from build123d import *

# Parameters (mm, degrees)
SKETCH1_W           = 80
SKETCH1_H           = 225
BOSS_EXTRUDE1_DEPTH = 29
CUT_EXTRUDE1_REACH  = 124.871
SKETCH4_R           = 10
CUT_EXTRUDE2_DEPTH  = 17
SKETCH5_R           = 8.5
CUT_EXTRUDE3_DEPTH  = 5
CUT_EXTRUDE4_REACH  = 124.871
SKETCH6_W           = 12
SKETCH6_H           = 11.5
M10_TAPPED_HOLE1_D  = 8.5
CUT_EXTRUDE5_REACH  = 124.871
SKETCH10_R          = 4


with BuildPart() as part:
    # Sketch1 → Boss-Extrude1 (new body)
    with BuildSketch(Plane(origin=(0, 0, 0), x_dir=(1, 0, 0), z_dir=(0, 1, 0))):
        Rectangle(SKETCH1_W, SKETCH1_H)
    extrude(amount=-BOSS_EXTRUDE1_DEPTH)

    # Sketch2 → Cut-Extrude1 (cut, up to next)
    with BuildSketch(Plane(origin=(0, 0, 0), x_dir=(1, 0, 0), z_dir=(0, 1, 0)), mode=Mode.PRIVATE) as cut_extrude1_sk1:
        with BuildLine():
            Line((-19, 36.36), (-19, 53.86))
            ThreePointArc((-19, 53.86), (-21.5, 56.36), (-24, 53.86))
            Line((-24, 53.86), (-24, 36.36))
            ThreePointArc((-24, 36.36), (-21.5, 33.86), (-19, 36.36))
        make_face()
    cut_extrude1_tool1 = extrude(cut_extrude1_sk1.sketch, amount=-CUT_EXTRUDE1_REACH, mode=Mode.PRIVATE) & part.part
    # Sketch2 → Cut-Extrude1 (cut, up to next)
    with BuildSketch(Plane(origin=(0, 0, 0), x_dir=(1, 0, 0), z_dir=(0, 1, 0)), mode=Mode.PRIVATE) as cut_extrude1_sk2:
        with BuildLine():
            Line((-19, -36.59), (-19, -16.59))
            ThreePointArc((-19, -16.59), (-21.5, -14.09), (-24, -16.59))
            Line((-24, -16.59), (-24, -36.59))
            ThreePointArc((-24, -36.59), (-21.5, -39.09), (-19, -36.59))
        make_face()
    cut_extrude1_tool2 = extrude(cut_extrude1_sk2.sketch, amount=-CUT_EXTRUDE1_REACH, mode=Mode.PRIVATE) & part.part
    # Sketch2 → Cut-Extrude1 (cut, up to next)
    with BuildSketch(Plane(origin=(0, 0, 0), x_dir=(1, 0, 0), z_dir=(0, 1, 0)), mode=Mode.PRIVATE) as cut_extrude1_sk3:
        with BuildLine():
            Line((24, 17.36), (24, 34.86))
            ThreePointArc((24, 34.86), (21.5, 37.36), (19, 34.86))
            Line((19, 34.86), (19, 17.36))
            ThreePointArc((19, 17.36), (21.5, 14.86), (24, 17.36))
        make_face()
    cut_extrude1_tool3 = extrude(cut_extrude1_sk3.sketch, amount=-CUT_EXTRUDE1_REACH, mode=Mode.PRIVATE) & part.part
    # Sketch2 → Cut-Extrude1 (cut, up to next)
    with BuildSketch(Plane(origin=(0, 0, 0), x_dir=(1, 0, 0), z_dir=(0, 1, 0)), mode=Mode.PRIVATE) as cut_extrude1_sk4:
        with BuildLine():
            Line((24, -36.64), (24, -12.64))
            ThreePointArc((24, -12.64), (21.5, -10.14), (19, -12.64))
            Line((19, -12.64), (19, -36.64))
            ThreePointArc((19, -36.64), (21.5, -39.14), (24, -36.64))
        make_face()
    cut_extrude1_tool4 = extrude(cut_extrude1_sk4.sketch, amount=-CUT_EXTRUDE1_REACH, mode=Mode.PRIVATE) & part.part
    add(cut_extrude1_tool1.solids().sort_by_distance((-21.5, 0, -45.11))[0], mode=Mode.SUBTRACT)
    add(cut_extrude1_tool2.solids().sort_by_distance((-21.5, 0, 26.59))[0], mode=Mode.SUBTRACT)
    add(cut_extrude1_tool3.solids().sort_by_distance((21.5, 0, -26.11))[0], mode=Mode.SUBTRACT)
    add(cut_extrude1_tool4.solids().sort_by_distance((21.5, 0, 24.64))[0], mode=Mode.SUBTRACT)

    # Sketch4 → Cut-Extrude2 (cut)
    with BuildSketch(Plane(origin=(0, 0, 0), x_dir=(1, 0, 0), z_dir=(0, 1, 0))):
        with Locations(Location((-22, 72, 0), (0, 0, 270))):
            Circle(SKETCH4_R)
        with Locations(Location((22, 60, 0), (0, 0, 270))):
            Circle(SKETCH4_R)
        with Locations(Location((0, 35, 0), (0, 0, 270))):
            Circle(SKETCH4_R)
        with Locations(Location((0, -25, 0), (0, 0, 270))):
            Circle(SKETCH4_R)
        with Locations(Location((22, -55, 0), (0, 0, 270))):
            Circle(SKETCH4_R)
        with Locations(Location((-22, -55, 0), (0, 0, 270))):
            Circle(SKETCH4_R)
    extrude(amount=-CUT_EXTRUDE2_DEPTH, mode=Mode.SUBTRACT)

    # Sketch5 → Cut-Extrude3 (cut)
    with BuildSketch(Plane.XZ.offset(29)):
        with Locations(Location((0, 100, 0), (0, 0, 270))):
            Circle(SKETCH5_R)
        with Locations(Location((0, -100, 0), (0, 0, 270))):
            Circle(SKETCH5_R)
    extrude(amount=-CUT_EXTRUDE3_DEPTH, mode=Mode.SUBTRACT)

    # Sketch6 → Cut-Extrude4 (cut, up to next)
    with BuildSketch(Plane(origin=(0, 0, 0), x_dir=(1, 0, 0), z_dir=(0, 1, 0)), mode=Mode.PRIVATE) as cut_extrude4_sk1:
        with Locations((23.25, -106.75)):
            Rectangle(SKETCH6_W, SKETCH6_H)
    cut_extrude4_tool1 = extrude(cut_extrude4_sk1.sketch, amount=-CUT_EXTRUDE4_REACH, mode=Mode.PRIVATE) & part.part
    add(cut_extrude4_tool1.solids().sort_by_distance((23.25, 0, 106.75))[0], mode=Mode.SUBTRACT)

    # M10 Tapped Hole1 (through all)
    with Locations(Plane(origin=(0, 0, 0), x_dir=(1, 0, 0), z_dir=(0, 1, 0))):
        with Locations((0, -77.5), (30, 4), (-30, 4), (0, 77.5)):
            Hole(M10_TAPPED_HOLE1_D / 2)

    # Sketch10 → Cut-Extrude5 (cut, up to next)
    with BuildSketch(Plane(origin=(0, 0, 0), x_dir=(1, 0, 0), z_dir=(0, 1, 0)), mode=Mode.PRIVATE) as cut_extrude5_sk1:
        with Locations(Location((0, 9.86, 0), (0, 0, 270))):
            Circle(SKETCH10_R)
    cut_extrude5_tool1 = extrude(cut_extrude5_sk1.sketch, amount=-CUT_EXTRUDE5_REACH, mode=Mode.PRIVATE) & part.part
    add(cut_extrude5_tool1.solids().sort_by_distance((0, 0, -9.86))[0], mode=Mode.SUBTRACT)


solid = part.part
Here's how the part is built. I have some questions about the finished solid (model axes, mm). A direction names the side the tool comes from. Coordinates: 2 decimals unless noted, no trailing zeros. Order: outer loops, then holes, each group sorted by start corner. A loop starts at its lowest first (then second) coordinate and runs counter-clockwise, first axis right, second up. Notation, with made-up numbers: M -12,-35.75 L 2,-35.75 A21 cw 2,-26.75 Z; hole C 51.25,58.25 d6. An arc over 180 degrees is marked long. Answer as CSV lines item,"result".
Item 1: For pin 1 (16 mm diameter, centred on x = -3, z = -40, fed in from +Y); pin 2 (7 mm diameter, centred on x = -30, z = -4, fed in from -Y); pin 3 (10 mm diameter, centred on x = 0, z = 100, fed in from -Y); pin 4 (6 mm diameter, centred on x = 20, z = -60, fed in from +Y), each with a flat end and sliding along its axis, tell me the tip position at first contact or that it passes through.
Results found:
pin 1,"y = 0"
pin 2,"through"
pin 3,"y = -24"
pin 4,"y = -17"
Item 2: Imagine slicing it at C-C on z = -60. Write out the boundary of the cut face in (x, y).
Results found:
outline,"M -40,-29 L 40,-29 L 40,0 L 32,0 L 32,-17 L 12,-17 L 12,0 L -40,0 Z"
Item 3: Imagine slicing it at A-A on y = -26.5. Give the number of separate pieces and of enclosed holes in the cut face, plus the area to 3 significant figures.
Results found:
separate pieces,"1"
enclosed holes,"11"
area,"16,700 mm2"
Item 4: On a 3-axis mill with a long thin cutter (end or side, diameter ignored), from which of +Z, -Z, +X, -X, +Y, -Y can I reach the whole of each face in a straight line? I mean faces 1 (the face through (-21.45, -14.3, 14.09)), 2 (the face through (0, -8, -45)), 3 (the face through (0.37, -26.54, -91.51)). Say none if no direction works.
Results found:
face 1,"+Y, -Y"
face 2,"+Y"
face 3,"-Y"
Item 5: We'd pull the mould along X, two halves only. Please class faces 4 (the face through (21.55, -14.3, -37.36)), 5 (the face through (-1, -29, -2)), 6 (the face through (-40, -14, 2)): +X half, -X half, draft (parallel to the pull), parting line (faces both ways), or undercut.
Results found:
face 4,"undercut"
face 5,"draft"
face 6,"-X half"
Item 6: Imagine slicing it at B-B on x = -30. Write out the boundary of the cut face in (y, z).
Results found:
outline,"M -29,-112.5 L 0,-112.5 L 0,-78 L -17,-78 L -17,-66 L 0,-66 L 0,-8.25 L -29,-8.25 Z; M -29,0.25 L 0,0.25 L 0,49 L -17,49 L -17,61 L 0,61 L 0,112.5 L -29,112.5 Z"
Item 7: If I drill on line 1 (X direction, y = -7.5, z = -49); line 2 (X direction, y = -8.5, z = -35); line 3 (Z direction, x = -27, y = -15), over which ranges is the centre line in solid material (lowest first)?
Results found:
line 1,"-40 to -24, -19 to 40"
line 2,"-40 to -23.6, -19.4 to -10, 10 to 19, 24 to 40"
line 3,"-112.5 to -80.66, -63.34 to -7.01, -0.99 to 46.34, 63.66 to 112.5"
